Autodesk Inventor part; units mm, degrees
ref_plane "Start Plane" through (0, 0, 0) normal (0, 0, 1) x (1, 0, 0)
ref_plane "End Plane" through (0, 0, 150) normal (0, 0, 1) x (1, 0, 0)
ref_plane "Work Plane4" through (0, 12.7, 150) normal (0.2991, 0, 0.9542) x (0.9542, 0, -0.2991)
ref_plane "Start Plane" through (0, 0, 0) normal (0, 0, 1) x (1, 0, 0)
ref_plane "End Plane" through (0, 0, 150) normal (0, 0, 1) x (1, 0, 0)
sketch "Sketch" plane through (0, 0, 0) normal (0, 0, 1) x (1, 0, 0)
  line L0 (25.4, 0) -> (0, 0)
  line L1 (0, 0) -> (0, 25.4)
  line L2 (0, 25.4) -> (1.651, 25.4)
  line L3 (3.175, 23.876) -> (3.175, 6.477)
  line L4 (6.477, 3.175) -> (23.876, 3.175)
  line L5 (25.4, 1.651) -> (25.4, 0)
  line L6 (0, -11.0414) -> (0, 31.5385) construction
  line L7 (-11.0414, 0) -> (31.5385, 0) construction
  arc A0 (3.175, 6.477) -> (6.477, 3.175) centre (6.477, 6.477) ccw
  arc A1 (3.175, 23.876) -> (1.651, 25.4) centre (1.651, 23.876) ccw
  arc A2 (25.4, 1.651) -> (23.876, 3.175) centre (23.876, 1.651) ccw
  line L8 (0, 40.0545) -> (0, -19.5574) construction
  line L9 (-19.5574, 0) -> (40.0545, 0) construction
  point P0 (3.175, 25.4)
  point P1 (3.175, 3.175)
  point P2 (25.4, 3.175)
  dimension "d0" = 25.4
  dimension "d1" = 25.4
  dimension "d2" = 3.175
  dimension "d3" = 3.175
  dimension "d10" = 0
  dimension "d11" = 0
  dimension "d14" = 3.302
  dimension "d15" = 1.524
extrude "Body" add sketch "Sketch" along normal up to surface (150 mm away) from surface at 0
sketch "Sketch3" plane through (0, 0, 0) normal (0, 0, 1) x (1, 0, 0)
  line L0 (0, 0) -> (10, 0)
ref_plane "Work Plane3" through (0, 0, 0) normal (0, -1, 0) x (1, 0, 0)
ref_plane "Work Plane4" through (0, 12.7, 150) normal (0.2991, 0, 0.9542) x (0.9542, 0, -0.2991)
split "Split1" plane through (0, 12.7, 150) removes the side toward (0.2991, 0, 0.9542)
ref_plane "Work Plane5" through (0, 690, 0) normal (0.8, 0, -0.6) x (-0.6, 0, -0.8)
split "Split2" plane through (0, 690, 0) removes the side toward (0.8, 0, -0.6)
sketch "Sketch4" plane through (0, 0, 0) normal (0, -1, 0) x (1, 0, 0)
  line L0 (-2, 0) -> (12, 0)
  line L1 (-2, 150) -> (12, 150)
  dimension "d17" = 150
equation "\"d0\" = G_H"
equation "\"d1\" = G_H"
equation "\"d2\" = G_T"
equation "\"d3\" = G_T"
equation "\"d14\" = G_IR"
equation "\"d15\" = G_ER"
equation "\"d4\" = G_L"
equation "\"G_H\" = 25.4"
equation "\"G_T\" = 3.175"
equation "\"G_ER\" = 1.524"
equation "\"G_IR\" = 3.302"
equation "\"G_L\" = d17"
equation "\"ex\" = 0"
equation "\"G_OFFSET_START\" = 0"
equation "\"G_OFFSET_END\" = 0"
equation "\"d13\" = G_OFFSET_END + B_L"
equation "\"B_L\" = 150"
properties part number "AISC - L 1 x 1 x 1/8 - 5.906" material "Steel, Mild"
Geometry: final body of the model. Coordinates: model frame, mm. A direction names the side the tool comes from. Coordinates: 2 decimals unless noted, no trailing zeros. Order: outer loops, then holes, each group sorted by start corner. A loop starts at its lowest first (then second) coordinate and runs counter-clockwise, first axis right, second up. Notation, with made-up numbers: M -7,45.5 L 29,45.5 A12 cw 29,49.5 Z; hole C -2.5,8 d7. An arc over 180 degrees is marked long. Answer in a Markdown table with one row per item. Add a question column.
Q1. Contact query for flat-ended pins moving along their axis: P1, Ø2, axis at y = 11.5, z = 124.5, coming from the -X side; P2, Ø14, axis at x = 12.5, z = 100, coming from the +Y side; P3, Ø8, axis at x = 8.5, z = 19, coming from the +Y side; P4, Ø12, axis at y = 16, z = 57.5, coming from the +X side (3 decimals). Output: stop coordinate, or through.
Q2. Section query A-A on z = 131. Return the cut outline in (x, y) (3 decimals).
Q3. Line query: L1, parallel to Y at x = 17, z = 127.5 (3 decimals); L2, parallel to X at y = 24.5, z = 95.5. Output: solid intervals per line, ascending.
Q4. Section query C-C on x = 21.25. Return the cut outline in (y, z) (3 decimals).
Q5. Reachability of faces 1 (the flat face through (0, 13, 74)), 2 (the flat face through (3.175, 15, 76)) from +Z, -Z, +X, -X, +Y, -Y: full face, straight path, thin tool, end or side. Return the list, or none.
Q6. Section query B-B on y = 8.5. Return the cut outline in (x, z) (3 decimals).
Q7. Section query D-D on z = 27.5. Return the cut outline in (x, y) (3 decimals).
Completed:
| question | item | result |
|---|---|---|
| 1 | P1 | stops at x = 0 |
| 1 | P2 | stops at y = 3.32 |
| 1 | P3 | stops at y = 3.83 |
| 1 | P4 | stops at x = 3.175 |
| 2 | outline | M 0,0 L 25.4,0 L 25.4,1.651 A1.524 ccw 23.876,3.175 L 6.477,3.175 A3.302 cw 3.175,6.477 L 3.175,23.876 A1.524 ccw 1.651,25.4 L 0,25.4 Z |
| 3 | L1 | y = 0 to 3.175 |
| 3 | L2 | x = 0 to 3.04 |
| 4 | outline | M 0,28.333 L 3.175,28.333 L 3.175,143.339 L 0,143.339 Z |
| 5 | face 1 | +Z, -Z, -X, +Y, -Y |
| 5 | face 2 | +Z, -Z, +X, +Y |
| 6 | outline | M 0,0 L 3.175,4.233 L 3.175,149.005 L 0,150 Z |
| 7 | outline | M 0,0 L 20.625,0 L 20.625,3.175 L 6.477,3.175 A3.302 cw 3.175,6.477 L 3.175,23.876 A1.524 ccw 1.651,25.4 L 0,25.4 Z |
